from build123d import *

# Parameters (mm, degrees)
EXTRUDE_1_DEPTH     = 1
EXTRUDE_2_DEPTH     = 4.8
SKETCH_4_W          = 2
SKETCH_4_H          = 5.8
EXTRUDE_3_DEPTH     = 10.45
SKETCH_5_W          = 2
SKETCH_5_H          = 2.95
EXTRUDE_4_DEPTH     = 1
SKETCH_6_W          = 2
SKETCH_6_H          = 1.5
CUT_EXTRUDE_1_DEPTH = 14.836274788
SKETCH_7_R          = 0.7
CUT_EXTRUDE_2_DEPTH = 16.122169157


with BuildPart() as part:
    # 草图1 → 凸台-拉伸1 (new body)
    with BuildSketch(Plane(origin=(0, 0, 0), x_dir=(1, 0, 0), z_dir=(0, 1, 0))):
        with BuildLine():
            Line((-4, 3.25), (-4, -4.25))
            Line((-4, -4.25), (4, -4.25))
            Line((4, -4.25), (4, 3.25))
            Line((4, 3.25), (2.1, 3.25))
            Line((2.1, 3.25), (2.1, 0))
            ThreePointArc((2.1, 0), (0, -2.1), (-2.1, 0))
            Line((-2.1, 0), (-2.1, 3.25))
            Line((-2.1, 3.25), (-4, 3.25))
        make_face()
    extrude(amount=EXTRUDE_1_DEPTH)

    # 草图3 → 凸台-拉伸2 (add)
    with BuildSketch(Plane(origin=(0, 1, 0), x_dir=(1, 0, 0), z_dir=(0, 1, 0))):
        Polygon((-3.3, 3.25), (-4, 3.25), (-4, -4.25), (4, -4.25), (4, 3.25), (3.3, 3.25), (3.3, -3.35), (-3.3, -3.35), align=None)
    extrude(amount=EXTRUDE_2_DEPTH)

    # 草图4 → 凸台-拉伸3 (add)
    with BuildSketch(Plane.XY.offset(4.25)):
        with Locations((5, 2.9)):
            Rectangle(SKETCH_4_W, SKETCH_4_H)
        with Locations((-5, 2.9)):
            Rectangle(SKETCH_4_W, SKETCH_4_H)
    extrude(amount=-EXTRUDE_3_DEPTH)

    # 草图5 → 凸台-拉伸4 (add)
    with BuildSketch(Plane(origin=(0, 5.8, 0), x_dir=(1, 0, 0), z_dir=(0, 1, 0))):
        Polygon((-6, 3.25), (-6, -4.25), (6, -4.25), (6, 3.25), (4, 3.25), (-4, 3.25), align=None)
        with Locations((-5, 4.725)):
            Rectangle(SKETCH_5_W, SKETCH_5_H)
        with Locations((5, 4.725)):
            Rectangle(SKETCH_5_W, SKETCH_5_H)
    extrude(amount=EXTRUDE_4_DEPTH)

    # 草图6 → 切除-拉伸1 (cut, through all)
    with BuildSketch(Plane.XY.offset(4.25)):
        with Locations((-2.1, 4.25)):
            Rectangle(SKETCH_6_W, SKETCH_6_H)
        with Locations((2.1, 4.25)):
            Rectangle(SKETCH_6_W, SKETCH_6_H)
    extrude(amount=-CUT_EXTRUDE_1_DEPTH, mode=Mode.SUBTRACT)

    # 草图7 → 切除-拉伸2 (cut, through all)
    with BuildSketch(Plane.ZY.offset(6)):
        with Locations(Location((-4.725, 5.3, 0), (0, 0, 270))):
            Circle(SKETCH_7_R)
        with Locations(Location((-4.725, 1.5, 0), (0, 0, 270))):
            Circle(SKETCH_7_R)
    extrude(amount=-CUT_EXTRUDE_2_DEPTH, mode=Mode.SUBTRACT)


solid = part.part
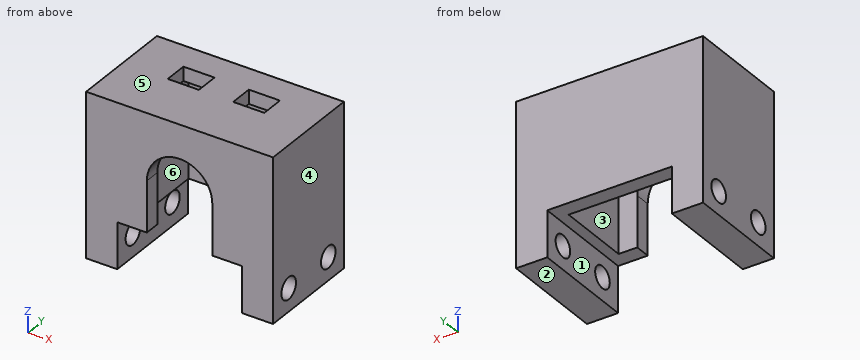
Model file for the job. Use its own axes, mm. Face numbers are marked on the shaded views. A direction names the side the tool comes from. Give positions to 0.01 mm unless a question says otherwise; leave off trailing zeros. Loops run counter-clockwise (first coordinate to the right, second up) from the corner with the lowest first, then second, coordinate; pieces in that order, holes last.
1) Saw through at B-B (z = 3). Write the cut outline in (x, y).
2) Tool access for the marked faces 5 and 6: list every direction of +Z, -Z, +X, -X, +Y, -Y with a clear straight run to the whole face (end or side of a thin tool).
3) Saw through at C-C (y = 1.5). Write the cut outline in (x, z) (3 decimals).
4) Flat gauge pins, fed straight in: pin 1 Ø2.5 at (x, y) = (-1, 4.5) entering from -Z; pin 2 Ø1.5 at (x, y) = (-3, 1) entering from -Z; pin 3 Ø0.8 at (y, z) = (5.3, -4.725) entering from -X. Where does each tip first touch, or does it go through?
5) Saw through at D-D (x = 0). Write the cut outline in (y, z), plus the area to 3 significant figures.
6) Wall check: line 1 (Y direction, x = 0.75, z = 3); line 2 (X direction, y = 2.25, z = -0.5); line 3 (Z direction, x = -5.25, y = 1.5) (3 decimals). Give the ranges that are in metal, low to high.
7) Saw through at A-A (x = 2.25). Write the cut outline in (y, z), plus the area to 3 significant figures.
8) Pull direction X, two halves, no side cores. Call the marked faces 1, 2, 3 and 4: +X half, -X half, draft (parallel to the pull), parting line (faces both ways), or undercut.
Answer block:
1. outline: (-6, 0) - (6, 0) - (6, 6.8) - (-6, 6.8) - close; hole (-3.3, 1) - (3.3, 1) - (3.3, 5.8) - (-3.3, 5.8) - close
2. face 5: +Z, +X, -X, +Y, -Y
2. face 6: -Z
3. outline: (-6, -6.2) - (-4, -6.2) - (-4, -5.425) - (-6, -5.425) - close; (-6, -4.025) - (-4, -4.025) - (-4, -3.25) - (-3.3, -3.25) - (-3.3, 3.35) - (3.3, 3.35) - (3.3, -3.25) - (4, -3.25) - (4, -4.025) - (6, -4.025) - (6, 4.25) - (-6, 4.25) - close; (4, -6.2) - (6, -6.2) - (6, -5.425) - (4, -5.425) - close
4. pin 1: stops at z = 3.35
4. pin 2: stops at z = -3.25
4. pin 3: passes through
5. outline: (0, 2.1) - (1, 2.1) - (1, 3.35) - (5.8, 3.35) - (5.8, -3.25) - (6.8, -3.25) - (6.8, 4.25) - (0, 4.25) - close
5. area: 14.0 mm2
6. line 1: y = 0 to 1, 5.8 to 6.8
6. line 2: x = -6 to -3.3, 3.3 to 6
6. line 3: z = -6.2 to -5.425, -4.025 to 4.25
7. outline: (0, -3.25) - (1, -3.25) - (1, 3.35) - (3.5, 3.35) - (3.5, 4.25) - (0, 4.25) - close; (5, 3.35) - (5.8, 3.35) - (5.8, -3.25) - (6.8, -3.25) - (6.8, 4.25) - (5, 4.25) - close
7. area: 18.0 mm2
8. face 1: undercut
8. face 2: draft
8. face 3: undercut
8. face 4: +X half
